Check sheet for the drawn part. Datum: minimum x, y, z corner. Units: mm. Give positions to 0.01 mm unless a question says otherwise; leave off trailing zeros. Loops run counter-clockwise (first coordinate to the right, second up) from the corner with the lowest first, then second, coordinate; pieces in that order, holes last. Notation, with made-up numbers: (11, 53) - (28, 53) arc R11 cw to (28, 61) - close; hole circle Ø2 at (27, -28). An arc over 180 degrees is marked (long way). Answer in a Markdown table with one row per item.
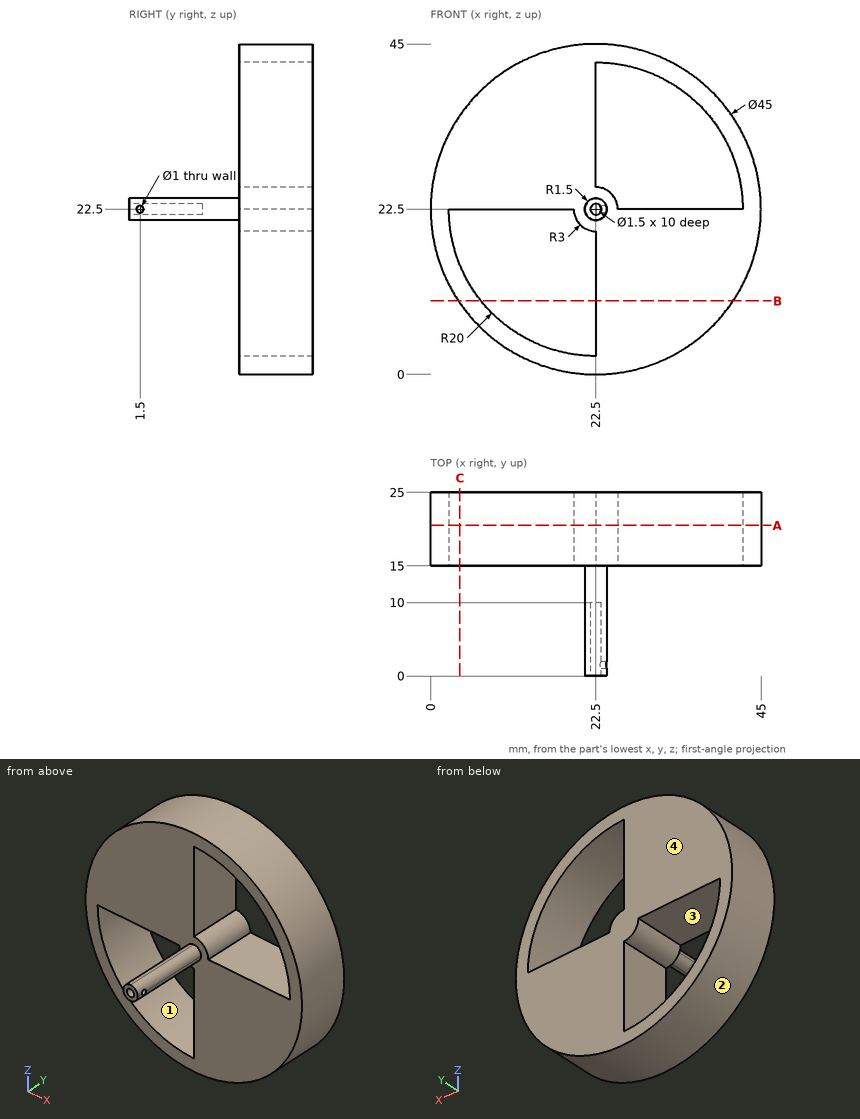
Q1. Thickness scan on line 1 (Y direction, x = 23.65, z = 22.5); line 2 (Z direction, x = 23.8, y = 1.5); line 3 (Y direction, x = 17, z = 32.5). Record the ranges inside material, lowest first.
Completed:
| item | result |
|---|---|
| line 1 | 0 to 1, 2 to 25 |
| line 2 | 21.75 to 22, 23 to 23.25 |
| line 3 | 15 to 25 |
Q2. Draft check along X on the marked faces 1, 2, 3 and 4. Enter one of: +X half, -X half, draft (parallel to the pull), parting line (faces both ways), or undercut.
Completed:
| item | result |
|---|---|
| face 1 | undercut |
| face 2 | parting line |
| face 3 | undercut |
| face 4 | draft |
Q3. Sectioned sample at B-B (z = 10). Record the cut outline in (x, y), and give its area (3 significant figures).
Completed:
| item | result |
|---|---|
| outline | (3.79, 15) - (6.89, 15) - (6.89, 25) - (3.79, 25) - close; (22.5, 15) - (41.21, 15) - (41.21, 25) - (22.5, 25) - close |
| area | 218 mm^2 |
Q4. Sectioned sample at A-A (y = 20.5). Record the cut outline in (x, z).
Completed:
| item | result |
|---|---|
| outline | circle Ø45 at (22.5, 22.5); hole (2.5, 22.5) arc R20 ccw to (22.5, 2.5) - (22.5, 19.5) arc R3 cw to (19.5, 22.5) - close; hole (22.5, 25.5) arc R3 cw to (25.5, 22.5) - (42.5, 22.5) arc R20 ccw to (22.5, 42.5) - close |
Q5. Sectioned sample at C-C (x = 4). Record the cut outline in (y, z).
Completed:
| item | result |
|---|---|
| outline | (15, 9.69) - (25, 9.69) - (25, 14.9) - (15, 14.9) - close; (15, 22.5) - (25, 22.5) - (25, 35.31) - (15, 35.31) - close |
Q6. Go/stop test with flat-tipped pins: P1, Ø5, axis at y = 19.5, z = 13, coming from the -X side; P2, Ø8, axis at x = 33.5, y = 20.5, coming from the +Z side; P3, Ø2, axis at x = 36, z = 33, coming from the -Y side; P4, Ø12, axis at x = 7.5, z = 6, coming from the -Y side. Record where each tip stops, or that it passes through.
Completed:
| item | result |
|---|---|
| P1 | x = 1.12 |
| P2 | z = 43.88 |
| P3 | through |
| P4 | y = 15 |
